Model file for the job. Use its own axes, mm. A direction names the side the tool comes from. Give positions to 0.01 mm unless a question says otherwise; leave off trailing zeros. Write each loop counter-clockwise with the first axis right and the second up, starting at its lowest first coordinate (ties: lowest second). Pieces come first, ordered by that corner, then holes.
```python
from build123d import *

# Parameters (mm, degrees)
BOSS_EXTRU_1_DEPTH = 10
CONG_1_R           = 0.3
CONG_2_R           = 0.5


with BuildPart() as part:
    # Esquisse1 → Boss.-Extru.1 (new body)
    with BuildSketch(Plane.XY):
        Polygon((10, 20.2), (18, 22.343593539), (18, 8.056406461), (10, 10.2), (10, 0), (0, 0), (0, 30.4), (10, 30.4), align=None)
    extrude(amount=BOSS_EXTRU_1_DEPTH)

    # Congé1
    cong_1_edges = [part.edges().sort_by_distance(p)[0] for p in [
        (14, 9.12820323, 0),
        (10, 5.1, 0),
        (5, 0, 0),
        (0, 15.2, 0),
        (10, 5.1, 10),
        (14, 9.12820323, 10),
        (18, 15.2, 10),
        (14, 21.27179677, 10),
        (10, 25.3, 10),
        (5, 30.4, 10),
        (0, 15.2, 10),
        (5, 30.4, 0),
        (5, 0, 10),
        (10, 25.3, 0),
        (14, 21.27179677, 0),
        (18, 15.2, 0),
    ]]
    fillet(cong_1_edges, radius=CONG_1_R)

    # Congé2
    # the kernel refuses this fillet: 0.5 mm, written as the material it takes off along each edge
    with BuildSketch(Plane(origin=(17.5, 21.691980853, 0), x_dir=(-0.25881904510251885, 0.9659258262890689, 0), z_dir=(-0.9659258262890689, -0.25881904510251885, 0))) as cong_2_piece_1:
        with BuildLine():
            CenterArc((0.2, -0.3), 0.3, 0, 90)
            Line((0.5, -0.3), (0.5, 0))
            Line((0.5, 0), (0.2, 0))
        make_face()
    revolve(axis=Axis((17.5, 21.691980853, 0), (0, 0, -1)), revolution_arc=105, mode=Mode.SUBTRACT)
    with BuildSketch(Plane(origin=(17.5, 8.708019147, 0), x_dir=(1, 0, 0), z_dir=(0, 1, 0))) as cong_2_piece_2:
        with BuildLine():
            CenterArc((0.2, -0.3), 0.3, 0, 90)
            Line((0.5, -0.3), (0.5, 0))
            Line((0.5, 0), (0.2, 0))
        make_face()
    revolve(axis=Axis((17.5, 8.708019147, 0), (0, 0, -1)), revolution_arc=105, mode=Mode.SUBTRACT)
    with BuildSketch(Plane(origin=(17.5, 8.708019147, 10), x_dir=(-0.25881904510251746, -0.9659258262890692, 0), z_dir=(-0.9659258262890692, 0.25881904510251746, 0))) as cong_2_piece_3:
        with BuildLine():
            CenterArc((0.2, -0.3), 0.3, 0, 90)
            Line((0.5, -0.3), (0.5, 0))
            Line((0.5, 0), (0.2, 0))
        make_face()
    revolve(axis=Axis((17.5, 8.708019147, 10), (0, 0, 1)), revolution_arc=105, mode=Mode.SUBTRACT)
    with BuildSketch(Plane(origin=(17.5, 21.691980853, 10), x_dir=(1, 0, 0), z_dir=(0, -1, 0))) as cong_2_piece_4:
        with BuildLine():
            CenterArc((0.2, -0.3), 0.3, 0, 90)
            Line((0.5, -0.3), (0.5, 0))
            Line((0.5, 0), (0.2, 0))
        make_face()
    revolve(axis=Axis((17.5, 21.691980853, 10), (0, 0, 1)), revolution_arc=105, mode=Mode.SUBTRACT)
    with BuildSketch(Plane(origin=(18, 8.056406461, 0), x_dir=(0, 1, 0), z_dir=(0, 0, 1)), Plane(origin=(18, 22.343593539, 0), x_dir=(-0.9659258262890698, -0.2588190451025152, 0), z_dir=(0, 0, 1))) as cong_2_piece_5:
        with BuildLine():
            CenterArc((CONG_2_R * 1.30322537284, CONG_2_R), CONG_2_R, 165, 105)
            Line((CONG_2_R * 0.337299546552, CONG_2_R * 1.2588190451), (0, 0))
            Line((0, 0), (CONG_2_R * 1.30322537284, 0))
        make_face()
    extrude(amount=10, mode=Mode.SUBTRACT)


solid = part.part
```
1. Pull direction X, two halves, no side cores. Call faces 5 (the flat face through (7, 15, 10)), 6 (the flat face through (13.737, 9.199, 4.934)), 7 (the flat face through (18, 15, 5)): +X half, -X half, draft (parallel to the pull), parting line (faces both ways), or undercut.
Calculated:
face 5: draft
face 6: undercut
face 7: +X half
2. Slice it at A-A, the plane y = 5. Write the cut outline in (x, z), and give its area (3 significant figures).
Calculated:
outline: (0, 0.3) arc R0.3 ccw to (0.3, 0) - (9.7, 0) arc R0.3 ccw to (10, 0.3) - (10, 9.7) arc R0.3 ccw to (9.7, 10) - (0.3, 10) arc R0.3 ccw to (0, 9.7) - close
area: 99.9 mm2
3. Probe probe 1 along X at (y, z) = (28.5, 4.75); probe 2 along Y at (x, z) = (16.75, 5.75). List the from-to ranges inside material, lowest first.
Calculated:
probe 1: x = 0 to 10
probe 2: y = 8.39 to 22.01
4. Which spindle directions (+Z, -Z, +X, -X, +Y, -Y) get a long thin tool onto all of the face, cutting with end or side? Do faces 1 (the cylindrical face through (13.57, 21.07, 0.09)), 2 (the cylindrical face through (13.46, 9.36, 9.91)), 3 (the flat face through (10, 5, 5)), 4 (the cylindrical face through (13.57, 21.07, 9.91)). Say none if no direction does.
Calculated:
face 1: -Z, +Y
face 2: +Z, -Y
face 3: +Z, -Z, -Y
face 4: +Z, +Y
5. Slice it at B-B, the plane z = 3. Write the cut outline in (x, y), and give its area (3 significant figures).
Calculated:
outline: (0, 0) - (10, 0) - (10, 10.2) - (17.37, 8.23) arc R0.5 ccw to (18, 8.71) - (18, 21.69) arc R0.5 ccw to (17.37, 22.17) - (10, 20.2) - (10, 30.4) - (0, 30.4) - close
area: 401 mm2
6. Pin check, flat tip, straight feed: P1, Ø4, axis at y = 26, z = 3.5, coming from the +X side. Stop position of the tip, or through.
Calculated:
P1: stops at x = 10
